```python
from build123d import *

# Parameters (mm, degrees)
CIRPATTERN1_COUNT = 6


with BuildPart() as part:
    # Sketch1 → Revolve1 (revolve)
    with BuildSketch(Plane.XY):
        with BuildLine():
            Line((-18.796, 53.975), (-10.16, 57.3024))
            Line((-10.16, 57.3024), (-0.508, 57.3024))
            Line((-0.508, 57.3024), (0, 57.16628181))
            Line((0, 57.16628181), (0, 51.69811819))
            Line((0, 51.69811819), (-0.508, 51.562))
            Line((-0.508, 51.562), (-12.954, 51.562))
            ThreePointArc((-12.954, 51.562), (-13.492815367, 51.338815367), (-13.716, 50.8))
            Line((-13.716, 50.8), (-13.716, 49.416677285))
            Line((-13.716, 49.416677285), (-14.478, 49.2125))
            Line((-14.478, 49.2125), (-26.416, 49.2125))
            Line((-26.416, 49.2125), (-26.416, 53.975))
            Line((-26.416, 53.975), (-18.796, 53.975))
        make_face()
    revolve(axis=Axis((0, 0, 0), (-1, 0, 0)))

    # Sketch6 → #6-32 Tapped Hole1 (revolve, cut)
    with BuildSketch(Plane(origin=(0, 0, 54.61), x_dir=(0, 0, -1), z_dir=(0, 1, 0))):
        Polygon((0, 0), (0, 9.70269403), (1.35255, 8.89), (1.35255, 0), align=None)
    f_6_32_tapped_hole1 = revolve(axis=Axis((6.35, 0, 54.61), (-1, 0, 0)), mode=Mode.SUBTRACT)

    # CirPattern1: #6-32 Tapped Hole1 ×6 about axis
    cirpattern1_axis = Axis((0, 0, 0), (1, 0, 0))
    for i in range(1, CIRPATTERN1_COUNT):
        add(f_6_32_tapped_hole1.rotate(cirpattern1_axis, i * 360 / CIRPATTERN1_COUNT), mode=Mode.SUBTRACT)


solid = part.part
```
Work out the finished part from the listing and answer in its coordinate system (mm). A direction names the side the tool comes from. Round coordinates to 2 decimals unless told otherwise and drop trailing zeros.
1) Consider probe 1 along Y at (x, z) = (-7.75, 0); probe 2 along Z at (x, y) = (-23.25, 0) (1 decimal); probe 3 along Y at (x, z) = (-18.75, 45.5). Determine where each line is inside the solid, lowest interval first.
2) Flat-ended cylindrical pins translate along their axes: P1, Ø1, axis at x = -5.5, y = -24.5, coming from the -Z side; P2, Ø2.5, axis at y = 0, z = -54.61, coming from the +X side; P3, Ø1, axis at x = -6.5, y = 14, coming from the -Z side. Find the tip coordinate at first contact, or state that the pin passes through.
3) Determine the mould class of faces 3 (the face through (0, -30, -43)), 4 (the face through (-9.562, -47.523, 27.254)), 5 (the face through (-22.55, -39.78, -36.48)) for opening direction Y: pulls with the +Y half, pulls with the -Y half, needs draft (parallel to the pull), parting line crosses it, or undercut.
4) Which of the six approach directions +Z, -Z, +X, -X, +Y, -Y give full straight-line access (tool end or side, diameter ignored) to faces 1 (the face through (-4.38, 0.06, -55.96)), 2 (the face through (-5.27, -12.42, 55.94))?
Entries:
1. probe 1: y = -57.3 to -51.56, 51.56 to 57.3
1. probe 2: z = -54 to -49.2, 49.2 to 54
1. probe 3: y = -29.07 to -18.75, 18.75 to 29.07
2. P1: stops at z = -52.03
2. P2: stops at x = -8.95
2. P3: stops at z = -55.69
3. face 3: needs draft
3. face 4: undercut
3. face 5: parting line crosses it
4. face 1: +X
4. face 2: +X, -X
